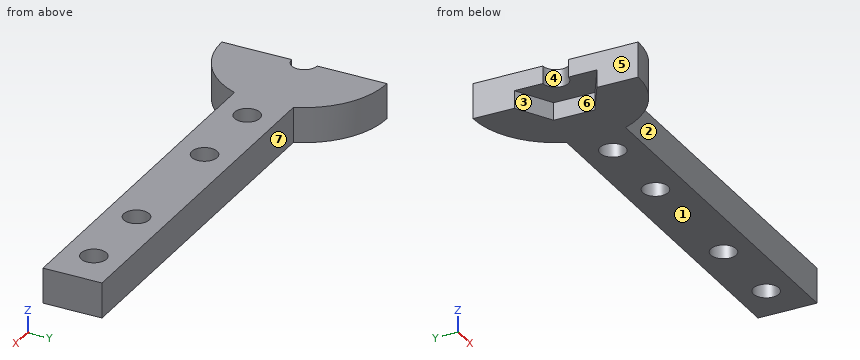
```python
from build123d import *

# Parameters (mm, degrees)
SKETCH_R     = 2.15
PAD_DEPTH    = 6
POCKET_DEPTH = 3


with BuildPart() as body:
    # Sketch → Pad (new body)
    with BuildSketch(Plane.XY):
        with BuildLine():
            Line((-13.076697, 5), (-75, 5))
            Line((-75, 5), (-75, -5))
            Line((-75, -5), (-13.076697, -5))
            ThreePointArc((-13.076697, -5), (-7.937254, -11.532563), (0, -14))
            Line((0, -2.15), (0, -14))
            ThreePointArc((0, 2.15), (-2.15, 0), (0, -2.15))
            Line((0, 14), (0, 2.15))
            ThreePointArc((0, 14), (-7.937254, 11.532563), (-13.076697, 5))
        make_face()
        with Locations((-68.1, 0)):
            Circle(SKETCH_R, mode=Mode.SUBTRACT)
        with Locations((-54.3, 0)):
            Circle(SKETCH_R, mode=Mode.SUBTRACT)
        with Locations((-32.3, 0)):
            Circle(SKETCH_R, mode=Mode.SUBTRACT)
        with Locations((-18.5, 0)):
            Circle(SKETCH_R, mode=Mode.SUBTRACT)
    extrude(amount=PAD_DEPTH)

    # Sketch001 → Pocket (cut)
    with BuildSketch(Plane.XY):
        Polygon((0, 7), (-6.062178, 3.5), (-6.062178, -3.5), (0, -7), align=None)
    extrude(amount=POCKET_DEPTH, mode=Mode.SUBTRACT)


with BuildPart() as part_mirroring:
    # Part__Mirroring: instance of Body
    add(body.part.mirror(Plane(origin=(0, 0, 0), x_dir=(0, -1, 0), z_dir=(1, 0, 0))))


solid = part_mirroring.part
```
Verification items for the finished model (mm, model axes). Face numbers are marked on the shaded views. A direction names the side the tool comes from. Give positions to 0.01 mm unless a question says otherwise; leave off trailing zeros. Loops run counter-clockwise (first coordinate to the right, second up) from the corner with the lowest first, then second, coordinate; pieces in that order, holes last. Notation, with made-up numbers: M -21.5,17.5 L -17.5,17.5 A7 ccw -17.5,24.5 Z; hole C 7,83 d10. An arc over 180 degrees is marked long. One line per question, with ' | ' between items.
Item 1: Draft check along Y on the marked faces 1, 2, 3 and 4. Enter one of: +Y half, -Y half, draft (parallel to the pull), parting line (faces both ways), or undercut.
Completed:
face 1: draft | face 2: -Y half | face 3: undercut | face 4: undercut
Item 2: Section check A-A, the plane y = 0. Record the cut outline in (x, z).
Completed:
outline: M 2.15,3 L 6.06,3 L 6.06,0 L 16.35,0 L 16.35,6 L 2.15,6 Z; M 20.65,0 L 30.15,0 L 30.15,6 L 20.65,6 Z; M 34.45,0 L 52.15,0 L 52.15,6 L 34.45,6 Z; M 56.45,0 L 65.95,0 L 65.95,6 L 56.45,6 Z; M 70.25,0 L 75,0 L 75,6 L 70.25,6 Z
Item 3: Depth check by flat-ended pin: P1, Ø3, axis at x = 41.5, z = 3, coming from the +Y side; P2, Ø3.5, axis at y = -1, z = 1, coming from the -X side. Enter the tip coordinate at first touch or a pass-through.
Completed:
P1: stops at y = 5 | P2: stops at x = 6.06
Item 4: Section check B-B, the plane z = 3.9. Record the cut outline in (x, y), plus the area to 3 significant figures.
Completed:
outline: M 0,-14 A14 ccw 13.08,-5 L 75,-5 L 75,5 L 13.08,5 A14 ccw 0,14 L 0,2.15 A2.15 cw 0,-2.15 Z; hole C 18.5,0 d4.3; hole C 32.3,0 d4.3; hole C 54.3,0 d4.3; hole C 68.1,0 d4.3 | area: 856 mm^2
Item 5: Section check C-C, the plane x = 54.3. Record the cut outline in (y, z), plus the area to 3 significant figures.
Completed:
outline: M -5,0 L -2.15,0 L -2.15,6 L -5,6 Z; M 2.15,0 L 5,0 L 5,6 L 2.15,6 Z | area: 34.2 mm^2
Item 6: Tool access check on the marked faces 5, 6 and 7. Record the directions out of +Z, -Z, +X, -X, +Y, -Y that give a thin tool (end or side, any length) a straight path to the whole face; none if there is none.
Completed:
face 5: +Z, -Z, -X, +Y, -Y | face 6: -Z, -X | face 7: +Z, -Z, +X, +Y
Item 7: Thickness scan on line 1 (Y direction, x = 54.3, z = 4.4); line 2 (X direction, y = 1, z = 1.25); line 3 (Y direction, x = 24.5, z = 5.6). Record the ranges inside material, lowest first. Write a range as [from, to].
Completed:
line 1: y = [-5, -2.15], [2.15, 5] | line 2: x = [6.06, 16.6], [20.4, 30.4], [34.2, 52.4], [56.2, 66.2], [70, 75] | line 3: y = [-5, 5]
Item 8: Section check D-D, the plane x = 15. Record the cut outline in (y, z).
Completed:
outline: M -5,0 L 5,0 L 5,6 L -5,6 Z
